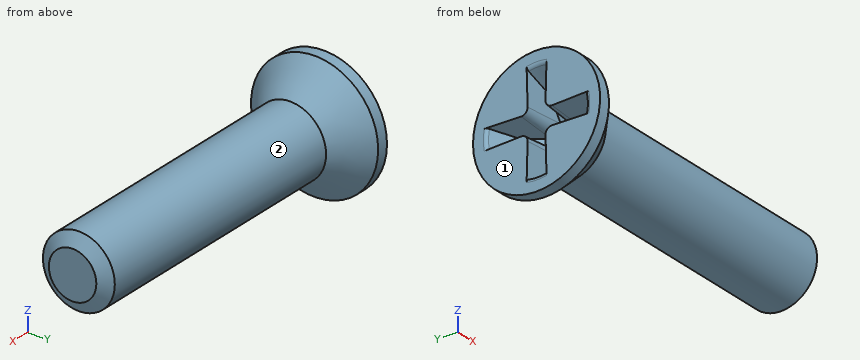
Autodesk Inventor part; units mm, degrees
ref_plane "Work Plane2" through (3.35, 0, 0) normal (0, 0, -1) x (1, 0, 0)
ref_plane "YZ Plane" through (0, 0, 0) normal (1, 0, 0) x (0, 1, 0)
ref_plane "XZ Plane" through (0, 0, 0) normal (0, 1, 0) x (-1, 0, 0)
sketch "Sketch1" plane through (0, 0, 0) normal (0, 0, 1) x (1, 0, 0)
  line L0 (2.3109, 0) -> (15.875, 0)
  line L1 (15.875, 0) -> (15.875, 1.7526)
  line L2 (15.875, 1.7526) -> (4.0926, 1.7526)
  line L3 (4.0926, 1.7526) -> (3.2988, 1.7526)
  line L4 (3.2988, 1.7526) -> (2.1082, 1.7526)
  line L5 (0, 3.0988) -> (0, 2.4765)
  line L6 (0, 2.4765) -> (1.3527, 1.8021)
  line L7 (1.3527, 1.8021) -> (2.3109, 0)
  line L8 (-3.175, 0) -> (19.05, 0)
  line L9 (0, -0.6198) -> (0, 3.7186)
  line L10 (0, 3.0988) -> (0.5596, 3.0988)
  line L11 (0.5596, 3.0988) -> (2.1082, 1.7526)
  line L12 (4.0926, 1.7526) -> (2.1082, 1.7526) construction
  dimension "d1" = 11.7824
  dimension "d2" = 3.5052
  dimension "d3" = 3.5052
  dimension "d4" = 4.953
  dimension "d5" = 26.5
  dimension "d6" = 62
  dimension "d7" = 2.3109
  dimension "d8" = 0.7937
  dimension "d12" = 6.1976
  dimension "d13" = 41
  dimension "d15" = 15.875
  dimension "d24" = 2.1082
revolve "Body" add sketch "Sketch1" angle 360 about axis through (2.3109, 0, 0) along (1, 0, 0) contours L7 L6 L5 L10 L11 L4 L3 L2 L1 L0
sketch "Sketch2" plane through (0, 0, 0) normal (-1, 0, 0) x (0, 0, 1)
  line L0 (0, 2.4765) -> (0, 0) construction
  line L1 (0, 0) -> (2.4765, 0) construction
  arc A0 (0.743, 0) -> (0, 0.7429) centre (0, 0) ccw construction
  arc A1 (0.8668, 0) -> (0, 0.8668) centre (0, 0) ccw construction
  arc A2 (2.429, 0.4826) -> (0.4826, 2.429) centre (0, 0) ccw
  line L2 (0, 0) -> (1.7511, 1.7511) construction
  line L3 (0.4826, 2.429) -> (0.4363, 0.749)
  line L4 (2.429, 0.4826) -> (0.749, 0.4363)
  arc A3 (0.4826, 2.429) -> (0, 2.4765) centre (0, 0) ccw
  arc A4 (2.4765, 0) -> (2.429, 0.4826) centre (0, 0) ccw
  line L5 (0, -4.3383) -> (0, 4.3383)
  line L6 (-4.3383, 0) -> (4.3383, 0)
  arc A5 (0.4826, -2.429) -> (2.429, -0.4826) centre (0, 0) ccw
  line L7 (0.4826, -2.429) -> (0.4363, -0.749)
  line L8 (2.429, -0.4826) -> (0.749, -0.4363)
  arc A6 (0, -2.4765) -> (0.4826, -2.429) centre (0, 0) ccw
  arc A7 (2.429, -0.4826) -> (2.4765, 0) centre (0, 0) ccw
  arc A8 (-0.4826, 2.429) -> (-2.429, 0.4826) centre (0, 0) ccw
  line L9 (-0.4826, 2.429) -> (-0.4363, 0.749)
  line L10 (-2.429, 0.4826) -> (-0.749, 0.4363)
  arc A9 (0, 2.4765) -> (-0.4826, 2.429) centre (0, 0) ccw
  arc A10 (-2.429, 0.4826) -> (-2.4765, 0) centre (0, 0) ccw
  arc A11 (-0.4826, -2.429) -> (0, -2.4765) centre (0, 0) ccw
  arc A12 (-2.429, -0.4826) -> (-0.4826, -2.429) centre (0, 0) ccw
  arc A13 (-2.4765, 0) -> (-2.429, -0.4826) centre (0, 0) ccw
  line L11 (-2.429, -0.4826) -> (-0.749, -0.4363)
  line L12 (-0.4826, -2.429) -> (-0.4363, -0.749)
  arc A14 (0.4363, 0.749) -> (0.749, 0.4363) centre (0.7406, 0.7406) ccw
  arc A15 (0.749, -0.4363) -> (0.4363, -0.749) centre (0.7406, -0.7406) ccw
  arc A16 (-0.749, 0.4363) -> (-0.4363, 0.749) centre (-0.7406, 0.7406) ccw
  arc A17 (-0.4363, -0.749) -> (-0.749, -0.4363) centre (-0.7406, -0.7406) ccw
  point P0 (1.7511, -1.7511)
  point P1 (-1.7511, 1.7511)
  point P2 (-1.7511, -1.7511)
  dimension "d17" = 1.4859
  dimension "d18" = 1.7335
  dimension "d19" = 4.953
  dimension "d20" = 45
  dimension "d21" = 0.4826
extrude "Slot" add sketch "Sketch2" against normal up to next draft 5 contours L4 A14 L3 A2 | A5 L7 A15 L8 | L9 A16 L10 A8 | A12 L11 A17 L12
fillet "Fillet1" radius 0.193 4 edges at (0, 2.4765, 0) (0, 0, -2.4765) (0, -2.4765, 0) (0, 0, 2.4765)
thread "Thread"
chamfer "Chamfer1" distance 0.5953 distance2 0.3969 1 edges at (15.875, -1.7526, 0) measured on face at (15.875, 0.1597, 0.4211)
ref_plane "Work Plane2" through (3.35, 0, 0) normal (0, 0, -1) x (1, 0, 0)
equation "\"d1\" = GEL"
equation "\"d2\" = GD"
equation "\"d3\" = BDM"
equation "\"d4\" = SDM"
equation "\"d7\" = INTI"
equation "\"d8\" = GAL"
equation "\"d12\" = KOD"
equation "\"d13\" = 0.5 * SEWI"
equation "\"d15\" = NLG"
equation "\"d24\" = KOH"
equation "\"d17\" = 0.3 * SDM"
equation "\"d18\" = 0.35 * SDM"
equation "\"d19\" = SDM"
equation "\"d21\" = 0.5 * SBR"
equation "\"d23\" = 0.2 * SBR"
equation "\"d10\" = GEL"
equation "\"d25\" = -0.5 * SPD + 0.5 * GD"
equation "\"d26\" = 0.5 * GAL"
equation "\"NLG\" = 15.875"
equation "\"GEL\" = 11.78242"
equation "\"GAL\" = 0.79375"
equation "\"SPD\" = 2.31458"
equation "\"KOD\" = 6.1976"
equation "\"KOH\" = 2.1082"
equation "\"SBR\" = 0.9652"
equation "\"SDM\" = 4.953"
equation "\"GD\" = NND"
equation "\"BDM\" = NND"
equation "\"SEWI\" = 82deg"
equation "\"d9\" = SDM"
equation "\"GUL\" = 0.75 * GAL"
equation "\"TOA\" = 30deg"
equation "\"THREADDIA\" = 3.5052"
equation "\"NND\" = 3.5052"
equation "\"INTI1\" = 2.8702"
equation "\"GD1\" = SPD"
properties part number "ANSI B18.6.3 - 6-32 x 5/8, CRFCHMSTII(3)" material "Steel, Mild"
Check sheet for the modelled part. Datum: model origin and axes. Units: mm. Face numbers are marked on the shaded views. A direction names the side the tool comes from. Coordinates: 2 decimals unless noted, no trailing zeros. Write each loop counter-clockwise with the first axis right and the second up, starting at its lowest first coordinate (ties: lowest second). Pieces come first, ordered by that corner, then holes. Notation, with made-up numbers: M 81,-33.5 L 110,-33.5 A30 cw 110,-7.5 Z; hole C 53.25,21.5 d10. An arc over 180 degrees is marked long. Answer as CSV lines item,"result".
Q1. Go/stop test with flat-tipped pins: pin 1 (1 mm diameter, centred on x = 8, y = 1, fed in from +Z); pin 2 (3 mm diameter, centred on x = 13.5, z = 2, fed in from +Y); pin 3 (1.5 mm diameter, centred on x = 11, y = 1.5, fed in from -Z). Record where each tip stops, or that it passes through.
Check result:
pin 1,"z = 1.68"
pin 2,"y = 1.68"
pin 3,"z = -1.58"
Q2. Material ranges on probe 1 along Z at (x, y) = (12.5, 0); probe 2 along Z at (x, y) = (13.75, 0.5); probe 3 along Y at (x, z) = (4.25, 1), recorded low to high. Write a range as from..to.
Check result:
probe 1,"-1.75..1.75"
probe 2,"-1.68..1.68"
probe 3,"-1.44..1.44"
Q3. Cross-section at A-A (x = 14.25). Record the boundary of the cut face in (y, z), then the cut area to 3 significant figures.
Check result:
outline,"C 0,0 d3.51"
area,"9.65 mm^2"
Q4. Set-up check for the marked faces 1 and 2: record each of +Z, -Z, +X, -X, +Y, -Y from which the full face is reachable in a straight line by a thin tool's end or side.
Check result:
face 1,"+Z, -Z, -X, +Y, -Y"
face 2,"+X"
